Job drawing, mm, ordinate dimensions from the low corner. One solid piece. A direction names the side the tool comes from. Round coordinates to 2 decimals unless told otherwise and drop trailing zeros. Write each loop counter-clockwise with the first axis right and the second up, starting at its lowest first coordinate (ties: lowest second). Pieces come first, ordered by that corner, then holes. Notation, with made-up numbers: M -12.75,34.5 L 2.25,34.5 A17 ccw 2.25,43.5 Z; hole C -37.75,-33 d1. An arc over 180 degrees is marked long. Write each question's results on one line, items separated by ' | '. Start each with the question number.
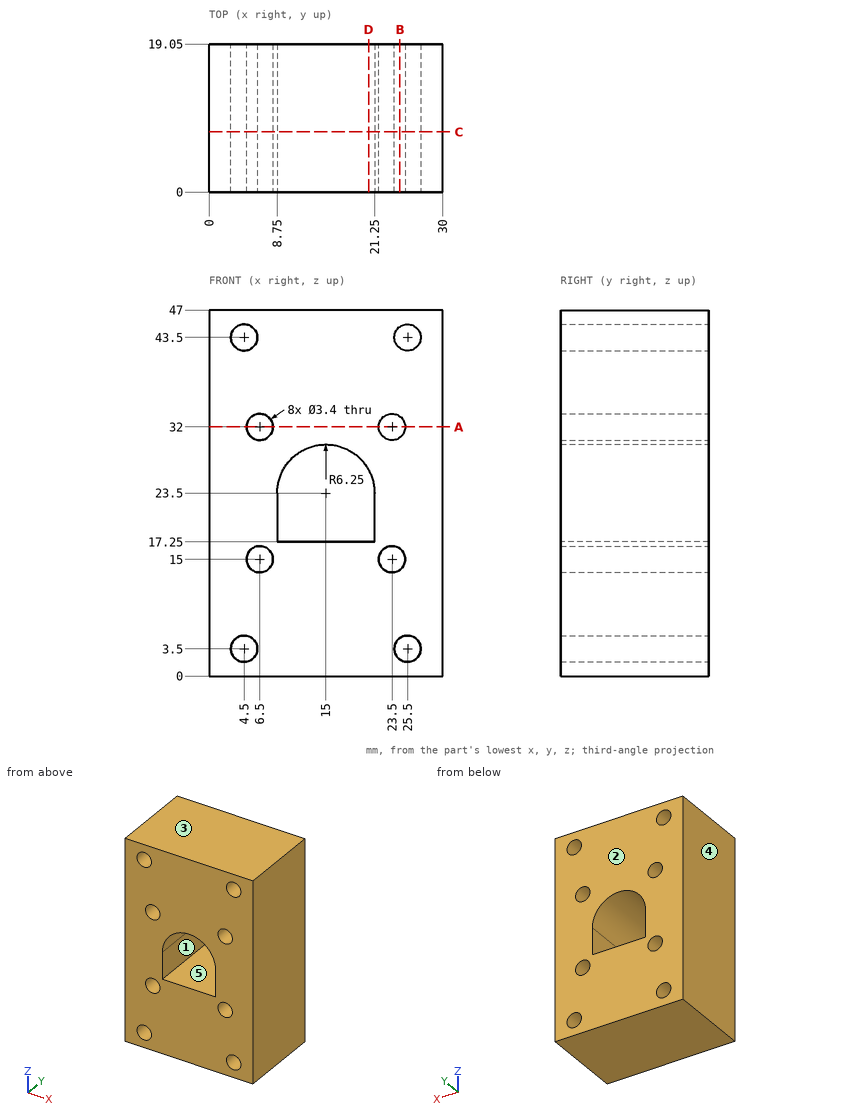
1) Saw through at A-A, the plane z = 32. Write the cut outline in (x, y), plus the area to 3 significant figures.
2) 3-axis set-ups, long thin cutter, end or side, ignore diameter. For the marked faces 1 and 2: which of +Z, -Z, +X, -X, +Y, -Y reach the whole face in a straight line?
3) Saw through at C-C, the plane y = 7.75. State how many separate pieces and enclosed holes the cut face has, plus the area to 3 significant figures.
4) Saw through at B-B, the plane x = 24.5. Write the cut outline in (y, z).
5) Pull direction Z, two halves, no side cores. Call the marked faces 3, 4 and 5: pulls with the +Z half, pulls with the -Z half, needs draft (parallel to the pull), parting line crosses it, or undercut.
6) Wall check: line 1 along X through (y, z) = (6, 15); line 2 along X through (y, z) = (12, 3.5); line 3 along Z through (x, y) = (23.5, 13.25). Give the ranges that are in metal, low to high. Write a range as from..to.
7) Drop a flat-ended pin along its axis: pin 1 Ø2 at (x, z) = (4.5, 43.5) entering from -Y (3 decimals). Give the stop position or say it passes through.
8) Saw through at D-D, the plane x = 20.5. Write the cut outline in (y, z), plus the area to 3 significant figures.
Filled sheet:
1) outline: M 0,0 L 4.8,0 L 4.8,19.05 L 0,19.05 Z; M 8.2,0 L 21.8,0 L 21.8,19.05 L 8.2,19.05 Z; M 25.2,0 L 30,0 L 30,19.05 L 25.2,19.05 Z | area: 442 mm^2
2) face 1: +Y, -Y | face 2: +Z, -Z, +X, -X, +Y
3) separate pieces: 1 | enclosed holes: 9 | area: 1,200 mm^2
4) outline: M 0,0 L 19.05,0 L 19.05,2.13 L 0,2.13 Z; M 0,4.87 L 19.05,4.87 L 19.05,13.63 L 0,13.63 Z; M 0,16.37 L 19.05,16.37 L 19.05,30.63 L 0,30.63 Z; M 0,33.37 L 19.05,33.37 L 19.05,42.13 L 0,42.13 Z; M 0,44.87 L 19.05,44.87 L 19.05,47 L 0,47 Z
5) face 3: pulls with the +Z half | face 4: needs draft | face 5: undercut
6) line 1: x = 0..4.8, 8.2..21.8, 25.2..30 | line 2: x = 0..2.8, 6.2..23.8, 27.2..30 | line 3: z = 0..13.3, 16.7..30.3, 33.7..47
7) pin 1: passes through
8) outline: M 0,0 L 19.05,0 L 19.05,17.25 L 0,17.25 Z; M 0,26.47 L 19.05,26.47 L 19.05,47 L 0,47 Z | area: 720 mm^2
